from build123d import *

# Parameters (mm, degrees)
CROQUIS1_R              = 200
CROQUIS1_R_2            = 150
CROQUIS1_R_3            = 5.4
SALIENTE_EXTRUIR1_DEPTH = 4


with BuildPart() as part:
    # Croquis1 → Saliente-Extruir1 (new body)
    with BuildSketch(Plane.XY):
        Circle(CROQUIS1_R)
        Circle(CROQUIS1_R_2, mode=Mode.SUBTRACT)
        with Locations((145.623058987, 105.801345413)):
            Circle(CROQUIS1_R_3, mode=Mode.SUBTRACT)
        with Locations((164.438182376, 73.212595754)):
            Circle(CROQUIS1_R_3, mode=Mode.SUBTRACT)
        with Locations((176.066568132, 37.424104347)):
            Circle(CROQUIS1_R_3, mode=Mode.SUBTRACT)
        with Locations((180, 0)):
            Circle(CROQUIS1_R_3, mode=Mode.SUBTRACT)
        with Locations((176.066568132, -37.424104347)):
            Circle(CROQUIS1_R_3, mode=Mode.SUBTRACT)
        with Locations((164.438182376, -73.212595754)):
            Circle(CROQUIS1_R_3, mode=Mode.SUBTRACT)
        with Locations((145.623058987, -105.801345413)):
            Circle(CROQUIS1_R_3, mode=Mode.SUBTRACT)
        with Locations((120.443509145, -133.766068586)):
            Circle(CROQUIS1_R_3, mode=Mode.SUBTRACT)
        with Locations((90, -155.884572681)):
            Circle(CROQUIS1_R_3, mode=Mode.SUBTRACT)
        with Locations((55.623058987, -171.190172933)):
            Circle(CROQUIS1_R_3, mode=Mode.SUBTRACT)
        with Locations((18.815123388, -179.013941166)):
            Circle(CROQUIS1_R_3, mode=Mode.SUBTRACT)
        with Locations((-18.815123388, -179.013941166)):
            Circle(CROQUIS1_R_3, mode=Mode.SUBTRACT)
        with Locations((-55.623058987, -171.190172933)):
            Circle(CROQUIS1_R_3, mode=Mode.SUBTRACT)
        with Locations((-90, -155.884572681)):
            Circle(CROQUIS1_R_3, mode=Mode.SUBTRACT)
        with Locations((-120.443509145, -133.766068586)):
            Circle(CROQUIS1_R_3, mode=Mode.SUBTRACT)
        with Locations((-145.623058987, -105.801345413)):
            Circle(CROQUIS1_R_3, mode=Mode.SUBTRACT)
        with Locations((-164.438182376, -73.212595754)):
            Circle(CROQUIS1_R_3, mode=Mode.SUBTRACT)
        with Locations((-176.066568132, -37.424104347)):
            Circle(CROQUIS1_R_3, mode=Mode.SUBTRACT)
        with Locations((-180, 0)):
            Circle(CROQUIS1_R_3, mode=Mode.SUBTRACT)
        with Locations((-176.066568132, 37.424104347)):
            Circle(CROQUIS1_R_3, mode=Mode.SUBTRACT)
        with Locations((-164.438182376, 73.212595754)):
            Circle(CROQUIS1_R_3, mode=Mode.SUBTRACT)
        with Locations((-145.623058987, 105.801345413)):
            Circle(CROQUIS1_R_3, mode=Mode.SUBTRACT)
        with Locations((-120.443509145, 133.766068586)):
            Circle(CROQUIS1_R_3, mode=Mode.SUBTRACT)
        with Locations((-90, 155.884572681)):
            Circle(CROQUIS1_R_3, mode=Mode.SUBTRACT)
        with Locations((-55.623058987, 171.190172933)):
            Circle(CROQUIS1_R_3, mode=Mode.SUBTRACT)
        with Locations((-18.815123388, 179.013941166)):
            Circle(CROQUIS1_R_3, mode=Mode.SUBTRACT)
        with Locations((18.815123388, 179.013941166)):
            Circle(CROQUIS1_R_3, mode=Mode.SUBTRACT)
        with Locations((55.623058987, 171.190172933)):
            Circle(CROQUIS1_R_3, mode=Mode.SUBTRACT)
        with Locations((90, 155.884572681)):
            Circle(CROQUIS1_R_3, mode=Mode.SUBTRACT)
        with Locations((120.443509145, 133.766068586)):
            Circle(CROQUIS1_R_3, mode=Mode.SUBTRACT)
    extrude(amount=SALIENTE_EXTRUIR1_DEPTH)


solid = part.part
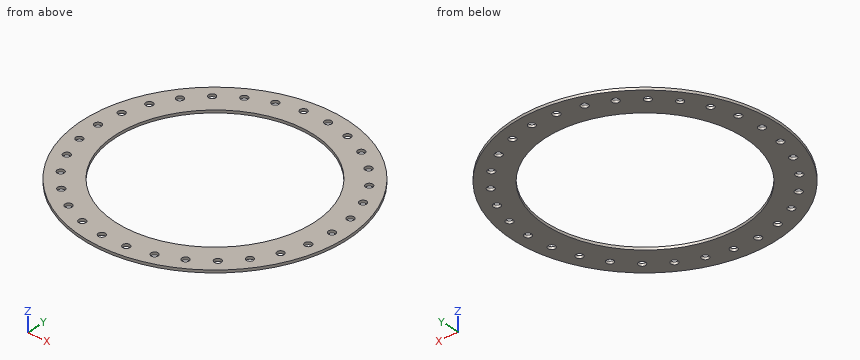
Design review of the part built by this model. Coordinates are the model's own, in mm. Give positions to 0.01 mm unless a question says otherwise; leave off trailing zeros. Loops run counter-clockwise (first coordinate to the right, second up) from the corner with the lowest first, then second, coordinate; pieces in that order, holes last. Notation, with made-up numbers: (73.5, 22.5) - (130.5, 22.5) arc R22 ccw to (130.5, 40.5) - close; hole circle Ø7 at (-36.5, 85). An arc over 180 degrees is marked (long way). Write item = value, one per line.
1) Take a section at A-A on y = 0. State the section outline as (x, z) points, and give its area (3 significant figures).
Result sheet:
outline = (-200, 0) - (-185.4, 0) - (-185.4, 4) - (-200, 4) - close; (-174.6, 0) - (-150, 0) - (-150, 4) - (-174.6, 4) - close; (150, 0) - (174.6, 0) - (174.6, 4) - (150, 4) - close; (185.4, 0) - (200, 0) - (200, 4) - (185.4, 4) - close
area = 314 mm2
2) To check wall thickness, follow line 1 (X direction, y = 104.5, z = 3.3); line 2 (Y direction, x = 22.5, z = 2.95); line 3 (X direction, y = 155, z = 0.7). State the ranges of each line that lie inside material, in increasing order.
Result sheet:
line_1 = -170.53 to -150.86, -140.38 to -107.61, 107.61 to 140.38, 150.86 to 170.53
line_2 = -198.73 to -182.96, -175.07 to -148.3, 148.3 to 175.07, 182.96 to 198.73
line_3 = -126.39 to -95.33, -84.67 to 84.67, 95.33 to 126.39
3) Take a section at C-C on z = 1.75. Count the separate pieces of the cut face and the enclosed holes in it, and give its area (3 significant figures).
Result sheet:
separate_pieces = 1
enclosed_holes = 31
area = 52,200 mm2
4) Take a section at D-D on y = 145. State the section outline as (x, z) points, and give its area (3 significant figures).
Result sheet:
outline = (-137.75, 0) - (-38.41, 0) - (-38.41, 4) - (-137.75, 4) - close; (38.41, 0) - (137.75, 0) - (137.75, 4) - (38.41, 4) - close
area = 795 mm2
5) Take a section at B-B on x = 0. State the section outline as (y, z) points.
Result sheet:
outline = (-200, 0) - (-150, 0) - (-150, 4) - (-200, 4) - close; (150, 0) - (200, 0) - (200, 4) - (150, 4) - close
6) Clearance check with flat-ended pins moving along their axes: pin 1 Ø2 at (y, z) = (-74, 2.5) entering from -X; pin 2 Ø2 at (x, z) = (-114.5, 3) entering from -Y. State where each tip first meets the part, or that it passes through.
Result sheet:
pin_1 = -186.2
pin_2 = -164.67
